Check sheet for the drawn part. Datum: minimum x, y, z corner. Units: mm. A direction names the side the tool comes from. Coordinates: 2 decimals unless noted, no trailing zeros. Loops run counter-clockwise (first coordinate to the right, second up) from the corner with the lowest first, then second, coordinate; pieces in that order, holes last.
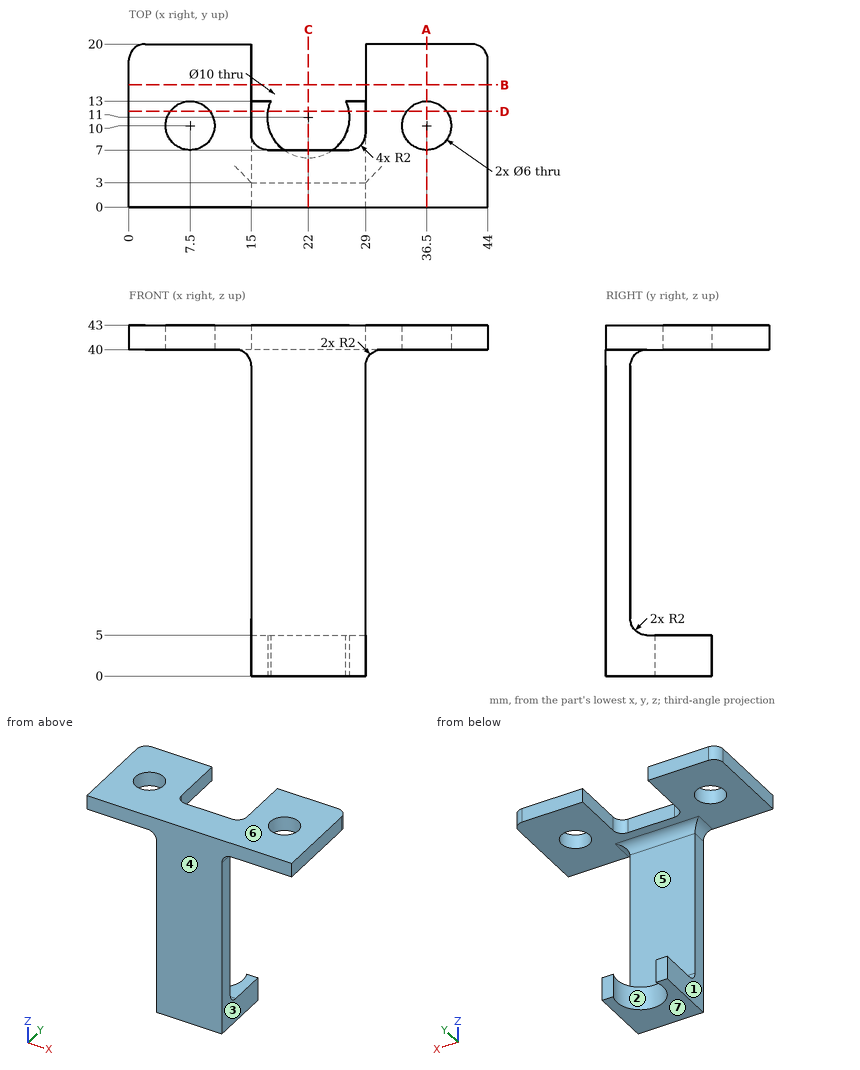
(1) Access from +Z, -Z, +X, -X, +Y, -Y to the whole of each face (thin tool, end or side, straight path). Record for the marked faces 1, 2 and 3.
Findings:
face 1: -Z, -X, +Y, -Y
face 2: -Z
face 3: -Z, +X, +Y, -Y
(2) Sectioned sample at C-C on x = 22. Record the cut outline in (y, z).
Findings:
outline: (0, 0) - (6, 0) - (6, 5) - (5, 5) arc R2 cw to (3, 7) - (3, 38) arc R2 cw to (5, 40) - (7, 40) - (7, 43) - (0, 43) - close
(3) Gauge pin test, flat ends, axial feed: pin 1 Ø2 at (x, y) = (5, 16.5) entering from -Z; pin 2 Ø15.5 at (x, z) = (20, 27) entering from +Y; pin 3 Ø6.5 at (y, z) = (6, 19) entering from -X. Record the tip position at first contact, or that the pin passes through.
Findings:
pin 1: stops at z = 40
pin 2: stops at y = 3
pin 3: stops at x = 15
(4) Draft check along Z on the marked faces 4, 5, 6 and 7. Enter one of: +Z half, -Z half, draft (parallel to the pull), parting line (faces both ways), or undercut.
Findings:
face 4: draft
face 5: undercut
face 6: +Z half
face 7: -Z half
(5) Sectioned sample at B-B on y = 15. Record the cut outline in (x, z), and give its area (3 significant figures).
Findings:
outline: (0, 40) - (15, 40) - (15, 43) - (0, 43) - close; (29, 40) - (44, 40) - (44, 43) - (29, 43) - close
area: 90.0 mm2
(6) Scan lines: L1, parallel to X at y = 11, z = 3.85; L2, parallel to Y at x = 22, z = 3; L3, parallel to Z at x = 11.5, y = 3.75. Record each from-to range of solid material in increasing order.
Findings:
L1: x = 15 to 17, 27 to 29
L2: y = 0 to 6
L3: z = 40 to 43
(7) Sectioned sample at A-A on x = 36.5. Record the cut outline in (y, z), and give its area (3 significant figures).
Findings:
outline: (0, 40) - (7, 40) - (7, 43) - (0, 43) - close; (13, 40) - (20, 40) - (20, 43) - (13, 43) - close
area: 42.0 mm2
(8) Sectioned sample at D-D on y = 11.75. Record the cut outline in (x, z), and give its area (3 significant figures).
Findings:
outline: (0, 40) - (5.06, 40) - (5.06, 43) - (0, 43) - close; (9.94, 40) - (15, 40) - (15, 43) - (9.94, 43) - close; (15, 0) - (17.06, 0) - (17.06, 5) - (15, 5) - close; (26.94, 0) - (29, 0) - (29, 5) - (26.94, 5) - close; (29, 40) - (34.06, 40) - (34.06, 43) - (29, 43) - close; (38.94, 40) - (44, 40) - (44, 43) - (38.94, 43) - close
area: 81.3 mm2
